```python
from build123d import *

# Parameters (mm, degrees)
BOSS_EXTRUDE1_DEPTH     = 10
SKETCH3_W               = 86
SKETCH3_H               = 8.65
SKETCH4_W               = 18
SKETCH4_H               = 18
BOSS_EXTRUDE2_DEPTH     = 10
SKETCH5_W               = 10
SKETCH5_H               = 10
CUT_EXTRUDE1_DEPTH      = 10
CUT_EXTRUDE1_DEPTH_BACK = 10
HOLE1_D                 = 4.134
HOLE1_DEPTH             = 9
HOLE1_CSINK_D           = 5
HOLE1_CSINK_ANGLE       = 90
HOLE2_D                 = 4.134
HOLE2_DEPTH             = 11
HOLE2_CSINK_D           = 5
HOLE2_CSINK_ANGLE       = 90
HOLE2_TIP               = 1.193383006


with BuildPart() as part:
    # Sketch1 → Revolve1 (revolve)
    with BuildSketch(Plane.XY):
        with BuildLine():
            Line((0, 0), (0, 7))
            Line((0, 7), (1, 8))
            Line((1, 8), (11.95, 8))
            Line((11.95, 8), (12.865685425, 7.084314575))
            ThreePointArc((12.865685425, 7.084314575), (13.125224104, 6.910896374), (13.43137085, 6.85))
            Line((13.43137085, 6.85), (14.2, 6.85))
            ThreePointArc((14.2, 6.85), (14.765685425, 7.084314575), (15, 7.65))
            Line((15, 7.65), (15, 8))
            Line((15, 8), (17, 8))
            Line((17, 8), (17, 0))
            Line((17, 0), (0, 0))
        make_face()
    revolve(axis=Axis((17, 0, 0), (-1, 0, 0)))

    # Sketch2 → Boss-Extrude1 (add)
    with BuildSketch(Plane(origin=(17, 0, 0), x_dir=(0, 0, -1), z_dir=(1, 0, 0))):
        with BuildLine():
            Line((-4.358898944, -9), (4.358898944, -9))
            ThreePointArc((4.358898944, -9), (7.071067812, -7.071067812), (9, -4.358898944))
            Line((9, -4.358898944), (9, 4.358898944))
            ThreePointArc((9, 4.358898944), (7.071067812, 7.071067812), (4.358898944, 9))
            Line((4.358898944, 9), (-4.358898944, 9))
            ThreePointArc((-4.358898944, 9), (-7.071067812, 7.071067812), (-9, 4.358898944))
            Line((-9, 4.358898944), (-9, -4.358898944))
            ThreePointArc((-9, -4.358898944), (-7.071067812, -7.071067812), (-4.358898944, -9))
        make_face()
    extrude(amount=BOSS_EXTRUDE1_DEPTH)

    # Sketch3 → Revolve2 (revolve)
    with BuildSketch(Plane.XY):
        with Locations((70, 4.325)):
            Rectangle(SKETCH3_W, SKETCH3_H)
    revolve(axis=Axis((113, 0, 0), (-1, 0, 0)))

    # Sketch4 → Boss-Extrude2 (add)
    with BuildSketch(Plane(origin=(113, 0, 0), x_dir=(0, 0, -1), z_dir=(1, 0, 0))):
        Rectangle(SKETCH4_W, SKETCH4_H)
    extrude(amount=BOSS_EXTRUDE2_DEPTH)

    # Sketch5 → Cut-Revolve1 (revolve, cut)
    with BuildSketch(Plane.XY):
        with Locations((118, 15)):
            Rectangle(SKETCH5_W, SKETCH5_H)
    revolve(axis=Axis((123, 0, 0), (-1, 0, 0)), mode=Mode.SUBTRACT)

    # Sketch6 → Revolve3 (revolve)
    with BuildSketch(Plane.XY):
        with BuildLine():
            Line((123, 0), (123, 8))
            Line((123, 8), (125, 8))
            Line((125, 8), (125, 7.65))
            ThreePointArc((125, 7.65), (125.234314575, 7.084314575), (125.8, 6.85))
            Line((125.8, 6.85), (126.56862915, 6.85))
            ThreePointArc((126.56862915, 6.85), (126.874775896, 6.910896374), (127.134314575, 7.084314575))
            Line((127.134314575, 7.084314575), (128.05, 8))
            Line((128.05, 8), (139, 8))
            Line((139, 8), (140, 7))
            Line((140, 7), (140, 0))
            Line((140, 0), (123, 0))
        make_face()
    revolve(axis=Axis((140, 0, 0), (-1, 0, 0)))

    # Sketch7 → Cut-Extrude1 (cut, two sides)
    with BuildSketch(Plane(origin=(0, 0, 0), x_dir=(1, 0, 0), z_dir=(0, 1, 0))) as cut_extrude1_sk:
        Polygon((118, 18), (118, 6), (140, 6), (140, -6), (118, -6), (118, -18), (152, -18), (152, 18), align=None)
    extrude(amount=CUT_EXTRUDE1_DEPTH, mode=Mode.SUBTRACT)
    extrude(cut_extrude1_sk.sketch, amount=-CUT_EXTRUDE1_DEPTH_BACK, mode=Mode.SUBTRACT)

    # Sketch8 → Cut-Revolve2 (revolve, cut)
    with BuildSketch(Plane(origin=(127, 0, 0), x_dir=(0, 0, -1), z_dir=(1, 0, 0))):
        Polygon((-6.2, 0), (-6.2, 4.692820323), (-5, 4), (-4.5, 4), (-5, 3.711324865), (-5, 3), (5, 3), (5, 3.711324865), (4.5, 4), (5, 4), (6.2, 4.692820323), (6.2, 0), align=None)
    revolve(axis=Axis((127, 0, -5), (0, 0, 1)), mode=Mode.SUBTRACT)

    # Hole1
    with Locations(Plane(origin=(0, 9, 0), x_dir=(1, 0, 0), z_dir=(0, 1, 0))):
        with Locations((23, 0)):
            CounterSinkHole(HOLE1_D / 2, HOLE1_CSINK_D / 2, depth=HOLE1_DEPTH, counter_sink_angle=HOLE1_CSINK_ANGLE)

    # Hole2
    with Locations(Plane(origin=(0, 9, 0), x_dir=(1, 0, 0), z_dir=(0, 1, 0))):
        with Locations((117, 0)):
            CounterSinkHole(HOLE2_D / 2, HOLE2_CSINK_D / 2, depth=HOLE2_DEPTH, counter_sink_angle=HOLE2_CSINK_ANGLE)
            with Locations((0, 0, -(HOLE2_DEPTH + HOLE2_TIP / 2))):  # 120° drill point
                Cone(0, HOLE2_D / 2, HOLE2_TIP, mode=Mode.SUBTRACT)

    # Sketch13 → Cut-Revolve3 (revolve, cut)
    with BuildSketch(Plane.XY):
        Polygon((-5, 0), (-5, 3), (41.2, 3), (41.2, 8), (95.2, 8), (95.2, 0), align=None)
    revolve(axis=Axis((95.2, 0, 0), (-1, 0, 0)), mode=Mode.SUBTRACT)


solid = part.part
```
The model under review builds one solid part; all positions refer to its coordinate system, in mm. A direction names the side the tool comes from. Round coordinates to 2 decimals unless told otherwise and drop trailing zeros. Order: outer loops, then holes, each group sorted by start corner. A loop starts at its lowest first (then second) coordinate and runs counter-clockwise, first axis right, second up. Notation, with made-up numbers: (68, 30) -> (81, 30) arc R17 ccw to (81, 34) -> close; hole circle Ø3 at (49.25, -36.5). An arc over 180 degrees is marked (long way). One line per item, written item: value. Start each with the question number.
Q1. Wall thickness on line 1 (X direction, y = 3.5, z = -7); line 2 (X direction, y = 0, z = 4.8); line 3 (X direction, y = -5.5, z = -7): over which ranges is each line inside the solid? List them lowest first.
Q2. Take a section at B-B (y = 0). Count the separate pieces of the cut face and the enclosed holes in it, and give its area (3 significant figures).
Q3. Machinability: for faces 1 (the face through (115.03, 3.21, -0.62)), 2 (the face through (118, 0, 7)), 3 (the face through (123, -8.4, 0.1)), 4 (the face through (113, -1.29, 8.71)), which of the approach directions +Z, -Z, +X, -X, +Y, -Y give a long, thin tool a straight path to every point of the face, cutting with its end or side? Answer none if there is none.
Q4. Take a section at A-A (x = 23). Write out the cut boundary in (y, z).
Q5. Clearance check with flat-ended pins moving along their axes: pin 1 Ø3 at (x, z) = (30, 2.5) entering from -Y; pin 2 Ø7 at (x, y) = (127, 0) entering from -Z; pin 3 Ø2.5 at (y, z) = (3.5, -8) entering from +X. State where each tip first meets the part, or that it passes through.
Q6. Take a section at D-D (x = 38.5). Write out the cut boundary in (y, z).
Q7. Mouldability with a two-part tool opening along Z and no side actions: class faces 5 (the face through (41.2, -3.4, -0.1)), 6 (the face through (6.55, -1.73, 7.81)), 7 (the face through (118, -9, 0)) as released by +Z, released by -Z, zero draft, split by the parting line, or undercut.
Q8. Take a section at C-C (x = 74). Write out the cut boundary in (y, z), and give its area (3 significant figures).
Reported:
1. line 1: x = 0.83 to 12.12, 15 to 41.2, 95.2 to 118
1. line 2: x = 0 to 41.2, 95.2 to 123, 123.17 to 124, 130 to 130.83, 131 to 140
1. line 3: x = 17 to 27, 113 to 118
2. separate pieces: 2
2. enclosed holes: 1
2. area: 1,090 mm2
3. face 1: +Y
3. face 2: +Z, +X, +Y, -Y
3. face 3: +X, -Y
3. face 4: none
4. outline: (-9, -4.36) arc R10 ccw to (-4.36, -9) -> (4.36, -9) arc R10 ccw to (9, -4.36) -> (9, -2.5) -> (8.57, -2.07) -> (2.17, -2.07) arc R3 cw (long way) to (2.17, 2.07) -> (8.57, 2.07) -> (9, 2.5) -> (9, 4.36) arc R10 ccw to (4.36, 9) -> (-4.36, 9) arc R10 ccw to (-9, 4.36) -> close
5. pin 1: stops at y = -8.59
5. pin 2: stops at z = -5
5. pin 3: stops at x = 118
6. outline: circle Ø17.3 at (0, 0); hole circle Ø6 at (0, 0)
7. face 5: undercut
7. face 6: split by the parting line
7. face 7: zero draft
8. outline: circle Ø17.3 at (0, 0); hole circle Ø16 at (0, 0)
8. area: 34.0 mm2
